The model under review builds one solid part; all positions refer to its coordinate system, in mm. A direction names the side the tool comes from. Give positions to 0.01 mm unless a question says otherwise; leave off trailing zeros. Order: outer loops, then holes, each group sorted by start corner. A loop starts at its lowest first (then second) coordinate and runs counter-clockwise, first axis right, second up. Notation, with made-up numbers: M 74,-14.5 L 133,-14.5 A31 cw 133,15.5 Z; hole C -17,-33 d11. An arc over 180 degrees is marked long. One line per question, with ' | ' between items. Start each with the question number.
1. The part is to be moulded in two halves that separate along X. For faces 1 (the face through (-1, 0, -0.75)), 2 (the face through (4, 0, -2)), 3 (the face through (-0.75, -0.03, 1.12)), 4 (the face through (-2.192, -5.916, -4.214)), say which applies: +X half, -X half, draft (parallel to the pull), parting line (faces both ways), or undercut.
2. For faces 5 (the face through (0, -6, -1)), 6 (the face through (-1.25, -5, 0)), 7 (the face through (0, -12, 0)), list the 3-axis set-ups (+Z, -Z, +X, -X, +Y, -Y) from which the entire face can be reached by the end or side of a thin tool; tool diameter is ignored.
3. We need section D-D on x = 2. Write out the cut boundary in (y, z).
4. We need section B-B on x = 0. Write out the cut boundary in (y, z), then the cut area to 4 significant figures.
5. Wall thickness on L1, parallel to Y at x = 0, z = 1.05; L2, parallel to Z at x = 0, y = -2.5; L3, parallel to X at y = -5.25, z = 0.5: over which ranges is each line inside the solid? List them lowest first.
6. We need section C-C on z = 0. Write out the cut boundary in (x, y), then the cut area to 3 significant figures.
7. We need section A-A on y = -1.5. Write out the cut boundary in (x, z), then the cut area to 3 significant figures.
8. Insertion check: P1, Ø3, axis at x = 1.5, z = 0, coming from the +Y side; P2, Ø0.6, axis at y = -4, z = -0.5, coming from the -X side; P3, Ø2, axis at y = -1, z = 2, coming from the -X side. Each pin has a flat end and moves straight along its axis. Give the tip position at first contact, or say it passes through.
Autodesk Inventor part; units mm, degrees
ref_plane "YZ Plane" through (0, 0, 0) normal (1, 0, 0) x (0, 1, 0)
ref_plane "XZ Plane" through (0, 0, 0) normal (0, 1, 0) x (-1, 0, 0)
ref_plane "XY Plane" through (0, 0, 0) normal (0, 0, 1) x (1, 0, 0)
sketch "Sketch1" plane through (0, 0, 0) normal (0, 1, 0) x (-1, 0, 0)
  circle A0 centre (0, 0) radius 4.75
  dimension "d0" = 9.5
extrude "Extrusion1" add sketch "Sketch1" against normal blind 12
sketch "Sketch2" plane through (0, 0, 0) normal (0, 1, 0) x (1, 0, 0)
  circle A0 centre (0, 0) radius 4
  dimension "d3" = 8
extrude "Extrusion2" cut sketch "Sketch2" against normal blind 10
sketch "Sketch3" plane through (0, 0, 0) normal (0, 0, 1) x (1, 0, 0)
  point P0 (0, 0)
sketch "Sketch4" plane through (0, 0, 0) normal (0, 0, 1) x (1, 0, 0)
  circle A0 centre (0, 0) radius 0.75
  circle A1 centre (0, 0) radius 1.25
  line L0 (-1.25, 0) -> (-1.25, -10)
  line L1 (-1.25, -10) -> (1.25, -10)
  line L2 (1.25, -10) -> (1.25, 0)
  dimension "d6" = 1.5
  dimension "d7" = 2.5
  dimension "d8" = 10
extrude "Extrusion3" add sketch "Sketch4" along normal mid plane 2 contours L2 L1 L0 A1
sketch "Sketch5" plane through (0, 0, 1) normal (0, 0, 1) x (1, 0, 0)
  circle A0 centre (0, 0) radius 0.75
  circle A1 centre (0, 0) radius 1.25
extrude "Extrusion4" add sketch "Sketch5" along normal mid plane 0.5
extrude "Extrusion5" add sketch "Sketch5" along normal blind 0.5
mirror "Mirror1" about plane through (0, 0, 0) normal (0, 0, 1) of "Extrusion4"
properties part number "Cylinder_1"
Entries:
1) face 1: undercut | face 2: draft | face 3: undercut | face 4: parting line
2) face 5: none | face 6: +Y | face 7: +Z, -Z, +X, -X, -Y
3) outline: M -12,-4.31 L 0,-4.31 L 0,-3.46 L -10,-3.46 L -10,3.46 L 0,3.46 L 0,4.31 L -12,4.31 Z
4) outline: M -12,-4.75 L 0,-4.75 L 0,-4 L -10,-4 L -10,-1 L -1.25,-1 L -1.25,-1.25 L -0.75,-1.25 L -0.75,-0.75 L -1.25,-0.75 L -1.25,0.75 L -0.75,0.75 L -0.75,1.5 L -1.25,1.5 L -1.25,1 L -10,1 L -10,4 L 0,4 L 0,4.75 L -12,4.75 Z; M 0.75,-1.25 L 1.25,-1.25 L 1.25,-0.75 L 0.75,-0.75 Z; M 0.75,0.75 L 1.25,0.75 L 1.25,1.5 L 0.75,1.5 Z | area: 52.75 mm^2
5) L1: y = -12 to -10, -1.25 to -0.75, 0.75 to 1.25 | L2: z = -4.75 to -4, -1 to 1, 4 to 4.75 | L3: x = -4.72 to -3.97, -1.25 to 1.25, 3.97 to 4.72
6) outline: M -4.75,-12 L 4.75,-12 L 4.75,0 L 4,0 L 4,-10 L 1.25,-10 L 1.25,0 A1.25 cw -1.25,0 L -1.25,-10 L -4,-10 L -4,0 L -4.75,0 Z | area: 56.5 mm^2
7) outline: C 0,0 d9.5; M -1.25,-1 L 1.25,-1 L 1.25,1 L -1.25,1 Z; hole C 0,0 d8 | area: 25.6 mm^2
8) P1: stops at y = 1.23 | P2: stops at x = -4.75 | P3: stops at x = -4.64
